from build123d import *

# Parameters (mm, degrees)
SKETCH_1_R               = 26
SKETCH_1_R_2             = 24
EXTRUDE_1_DEPTH          = 194
SKETCH_2_R               = 1.5
CUT_EXTRUDE_1_DEPTH      = 88
PATTERN_CIRCULAR_1_COUNT = 3
SKETCH_3_W               = 5
SKETCH_3_H               = 11.473941433
CUT_EXTRUDE_2_DEPTH      = 2
PATTERN_CIRCULAR_2_COUNT = 3
SKETCH_4_W               = 5
SKETCH_4_H               = 11.473941433
CUT_EXTRUDE_3_DEPTH      = 2
PATTERN_CIRCULAR_3_COUNT = 3


with BuildPart() as part:
    # Эскиз1 → Бобышка-Вытянуть1 (new body)
    with BuildSketch(Plane.XY):
        with Locations(Location((0, 0, 0), (0, 0, 180))):
            Circle(SKETCH_1_R)
        with Locations(Location((0, 0, 0), (0, 0, 180))):
            Circle(SKETCH_1_R_2, mode=Mode.SUBTRACT)
    extrude(amount=EXTRUDE_1_DEPTH)

    # Эскиз2 → Вырез-Вытянуть1 (cut)
    with BuildSketch(Plane(origin=(0, 0, 0), x_dir=(1, 0, 0), z_dir=(0, 1, 0))):
        with Locations(Location((0, -5, 0), (0, 0, 270))):
            Circle(SKETCH_2_R)
        with Locations(Location((0, -189, 0), (0, 0, 270))):
            Circle(SKETCH_2_R)
    cut_extrude_1 = extrude(amount=-CUT_EXTRUDE_1_DEPTH, mode=Mode.SUBTRACT)

    # Круговой массив1: Вырез-Вытянуть1 ×3 about axis
    pattern_circular_1_axis = Axis((0, 0, 194), (0, 0, -1))
    for i in range(1, PATTERN_CIRCULAR_1_COUNT):
        add(cut_extrude_1.rotate(pattern_circular_1_axis, i * 360 / PATTERN_CIRCULAR_1_COUNT), mode=Mode.SUBTRACT)

    # Эскиз3 → Вырез-Вытянуть2 (cut)
    with BuildSketch(Plane(origin=(0, 0, 0), x_dir=(-1, 0, 0), z_dir=(0, 0, -1))):
        with Locations((0, 22.870937025)):
            Rectangle(SKETCH_3_W, SKETCH_3_H)
    cut_extrude_2 = extrude(amount=-CUT_EXTRUDE_2_DEPTH, mode=Mode.SUBTRACT)

    # Круговой массив2: Вырез-Вытянуть2 ×3 about axis
    pattern_circular_2_axis = Axis((0, 0, 0), (0, 0, 1))
    for i in range(1, PATTERN_CIRCULAR_2_COUNT):
        add(cut_extrude_2.rotate(pattern_circular_2_axis, i * 360 / PATTERN_CIRCULAR_2_COUNT), mode=Mode.SUBTRACT)

    # Эскиз4 → Вырез-Вытянуть3 (cut)
    with BuildSketch(Plane.XY.offset(194)):
        with Locations((0, 22.870937025)):
            Rectangle(SKETCH_4_W, SKETCH_4_H)
    cut_extrude_3 = extrude(amount=-CUT_EXTRUDE_3_DEPTH, mode=Mode.SUBTRACT)

    # Круговой массив3: Вырез-Вытянуть3 ×3 about axis
    pattern_circular_3_axis = Axis((0, 0, 0), (0, 0, 1))
    for i in range(1, PATTERN_CIRCULAR_3_COUNT):
        add(cut_extrude_3.rotate(pattern_circular_3_axis, i * 360 / PATTERN_CIRCULAR_3_COUNT), mode=Mode.SUBTRACT)


solid = part.part
Design review of the part built by this model. Coordinates are the model's own, in mm. A direction names the side the tool comes from. Give positions to 0.01 mm unless a question says otherwise; leave off trailing zeros. Order: outer loops, then holes, each group sorted by start corner. A loop starts at its lowest first (then second) coordinate and runs counter-clockwise, first axis right, second up. Notation, with made-up numbers: (82, 7) - (96, 7) arc R34 ccw to (96, 37) - close; hole circle Ø8 at (33, -19.75). An arc over 180 degrees is marked (long way). Write item = value, one per line. Start each with the question number.
Q1. Mouldability with a two-part tool opening along Z and no side actions: class faces 4 (the face through (0.1, -24.5, 194)), 5 (the face through (21.906, 11.984, 190.386)), 6 (the face through (0.1, -24.5, 0)) as released by +Z, released by -Z, zero draft, split by the parting line, or undercut.
Q2. We need section B-B on x = -7. State the section outline as (y, z) points, plus the area to 3 significant figures.
Q3. We need section C-C on z = 152. State the section outline as (x, y) points.
Q4. We need section A-A on y = 0. State the section outline as (x, z) points.
Q5. Tool access review of faces 1 (the face through (-22, -12, 2)), 2 (the face through (22, -12, 192)), 3 (the face through (21.39, 12.87, 6.43)): name each direction out of +Z, -Z, +X, -X, +Y, -Y from which nothing blocks a thin tool from reaching the whole face with its end or side.
Q6. To check wall thickness, follow L1, parallel to Y at x = -1, z = 73; L2, parallel to Z at x = 0, y = -25.45; L3, parallel to X at y = 13.5, z = 157. State the ranges of each line that lie inside material, in increasing order. Write a range as from..to.
Q7. Clearance check with flat-ended pins moving along their axes: pin 1 Ø3.5 at (x, y) = (-21.5, -12) entering from -Z; pin 2 Ø2.5 at (x, y) = (-1, 25.5) entering from +Z; pin 3 Ø5 at (x, z) = (7, 148) entering from +Y. State where each tip first meets the part, or that it passes through.
Working result:
q1.face_4 = released by +Z
q1.face_5 = undercut
q1.face_6 = released by -Z
q2.outline = (-25.04, 0) - (-22.96, 0) - (-22.96, 194) - (-25.04, 194) - close; (22.96, 0) - (25.04, 0) - (25.04, 194) - (22.96, 194) - close
q2.area = 808 mm²
q3.outline = circle Ø52 at (0, 0); hole circle Ø48 at (0, 0)
q4.outline = (-26, 0) - (-24, 0) - (-24, 194) - (-26, 194) - close; (24, 0) - (26, 0) - (26, 194) - (24, 194) - close
q5.face_1 = -Z
q5.face_2 = +Z
q5.face_3 = none
q6.L1 = -25.98..-23.98, 23.98..25.98
q6.L2 = 0..3.5, 6.5..187.5, 190.5..194
q6.L3 = -22.22..-19.84, 19.84..22.22
q7.pin_1 = 2
q7.pin_2 = 192
q7.pin_3 = 25.61
